Geometry check sheet. Reference: the model listing, model coordinates, mm. Face numbers are marked on the shaded views. A direction names the side the tool comes from. Coordinates: 2 decimals unless noted, no trailing zeros. Loops run counter-clockwise (first coordinate to the right, second up) from the corner with the lowest first, then second, coordinate; pieces in that order, holes last.
from build123d import *

# Parameters (mm, degrees)
SKETCH_1_W          = 30
SKETCH_1_H          = 13
EXTRUDE_1_DEPTH     = 1.4
SKETCH_2_W          = 30
SKETCH_2_H          = 13
EXTRUDE_2_DEPTH     = 4
SKETCH_3_W          = 30
SKETCH_3_H          = 13
EXTRUDE_3_DEPTH     = 1.6
SKETCH_4_W          = 30
SKETCH_4_H          = 8.5
EXTRUDE_4_DEPTH     = 4.5
SKETCH_6_W          = 16.5
SKETCH_6_H          = 7.2
SKETCH_6_W_2        = 15.3
SKETCH_6_H_2        = 6
SKETCH_6_W_3        = 7.5
SKETCH_6_R          = 3
EXTRUDE_5_DEPTH     = 2
SKETCH_7_W          = 10.5
SKETCH_7_H          = 4.5
CUT_EXTRUDE_1_DEPTH = 12
SKETCH_8_W          = 10
SKETCH_8_H          = 1.1
EXTRUDE_6_DEPTH     = 8.05


with BuildPart() as part:
    # Эскиз1 → Бобышка-Вытянуть1 (new body)
    with BuildSketch(Plane.XY):
        with Locations((0, 6.5)):
            Rectangle(SKETCH_1_W, SKETCH_1_H)
    extrude(amount=EXTRUDE_1_DEPTH)

    # Эскиз2 → Бобышка-Вытянуть2 (add)
    with BuildSketch(Plane.XY.offset(1.4)):
        with Locations((0, 6.5)):
            Rectangle(SKETCH_2_W, SKETCH_2_H)
    extrude(amount=EXTRUDE_2_DEPTH)

    # Эскиз3 → Бобышка-Вытянуть3 (add)
    with BuildSketch(Plane.XY.offset(5.4)):
        with Locations((0, 6.5)):
            Rectangle(SKETCH_3_W, SKETCH_3_H)
    extrude(amount=EXTRUDE_3_DEPTH)

    # Эскиз4 → Бобышка-Вытянуть4 (add)
    with BuildSketch(Plane.XY.offset(7)):
        with Locations((0, 6.5)):
            Rectangle(SKETCH_4_W, SKETCH_4_H)
    extrude(amount=EXTRUDE_4_DEPTH)

    # Эскиз6 → Бобышка-Вытянуть5 (add)
    # profile 1 of 2: a face of its own
    with BuildSketch(Plane.XY.offset(11.5)):
        with Locations((5.95, 6.5)):
            Rectangle(SKETCH_6_W, SKETCH_6_H)
        with Locations((5.95, 6.5)):
            Rectangle(SKETCH_6_W_2, SKETCH_6_H_2, mode=Mode.SUBTRACT)
    # profile 2 of 2: a face of its own
    with BuildSketch(Plane.XY.offset(11.5)):
        with Locations((-10.45, 6.5)):
            Rectangle(SKETCH_6_W_3, SKETCH_6_H)
        with Locations((-10.45, 6.5)):
            Circle(SKETCH_6_R, mode=Mode.SUBTRACT)
    extrude(amount=EXTRUDE_5_DEPTH)

    # Эскиз7 → Вырез-Вытянуть1 (cut)
    with BuildSketch(Plane.XY.offset(7)):
        Rectangle(SKETCH_7_W, SKETCH_7_H)
    extrude(amount=-CUT_EXTRUDE_1_DEPTH, mode=Mode.SUBTRACT)

    # Эскиз8 → Бобышка-Вытянуть6 (add)
    with BuildSketch(Plane.XZ.offset(-2.25)):
        with Locations((0, 3.05)):
            Rectangle(SKETCH_8_W, SKETCH_8_H)
    extrude(amount=EXTRUDE_6_DEPTH)


solid = part.part
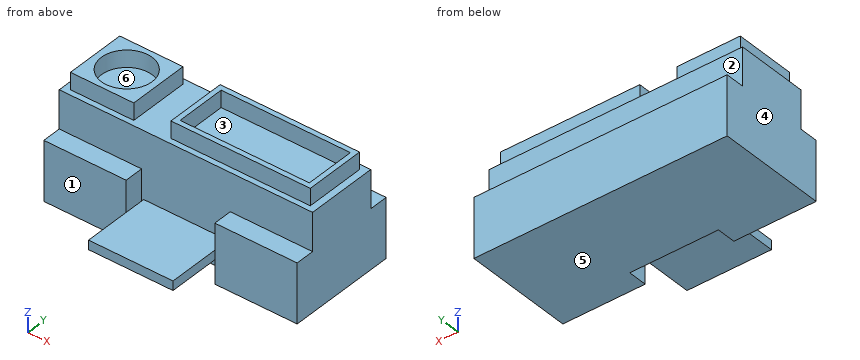
(1) Access from +Z, -Z, +X, -X, +Y, -Y to the whole of each face (thin tool, end or side, straight path). Record for the marked faces 1, 2 and 3.
Findings:
face 1: +Z, -Z, -X, -Y
face 2: +Z, +X, -X, +Y
face 3: +Z
(2) Sectioned sample at B-B on y = 6.5. Record the cut outline in (x, z), and give its area (3 significant figures).
Findings:
outline: (-15, 0) - (15, 0) - (15, 11.5) - (14.2, 11.5) - (14.2, 13.5) - (13.6, 13.5) - (13.6, 11.5) - (-1.7, 11.5) - (-1.7, 13.5) - (-2.3, 13.5) - (-2.3, 11.5) - (-6.7, 11.5) - (-6.7, 13.5) - (-7.45, 13.5) - (-7.45, 11.5) - (-13.45, 11.5) - (-13.45, 13.5) - (-14.2, 13.5) - (-14.2, 11.5) - (-15, 11.5) - close
area: 350 mm2
(3) Sectioned sample at D-D on x = -12.5. Record the cut outline in (y, z).
Findings:
outline: (0, 0) - (13, 0) - (13, 7) - (10.75, 7) - (10.75, 11.5) - (10.1, 11.5) - (10.1, 13.5) - (8.69, 13.5) - (8.69, 11.5) - (4.31, 11.5) - (4.31, 13.5) - (2.9, 13.5) - (2.9, 11.5) - (2.25, 11.5) - (2.25, 7) - (0, 7) - close
(4) Scan lines: L1, parallel to Y at x = -10.45, z = 12.2; L2, parallel to Z at x = -6.25, y = 12; L3, parallel to Z at x = 4.5, y = 10.5. Record each from-to range of solid material in increasing order.
Findings:
L1: y = 2.9 to 3.5, 9.5 to 10.1
L2: z = 0 to 7
L3: z = 0 to 11.5
(5) Gauge pin test, flat ends, axial feed: pin 1 Ø1.6 at (x, z) = (5.5, 12.5) entering from +Y; pin 2 Ø1.5 at (x, y) = (-0.5, 8.5) entering from +Z; pin 3 Ø1.6 at (y, z) = (5, 13) entering from -X. Record the tip position at first contact, or that the pin passes through.
Findings:
pin 1: stops at y = 10.1
pin 2: stops at z = 11.5
pin 3: stops at x = -14.2
(6) Sectioned sample at A-A on z = 6. Record the cut outline in (x, y), and give its area (3 significant figures).
Findings:
outline: (-15, 0) - (-5.25, 0) - (-5.25, 2.25) - (5.25, 2.25) - (5.25, 0) - (15, 0) - (15, 13) - (-15, 13) - close
area: 366 mm2
(7) Sectioned sample at C-C on x = 9.5. Record the cut outline in (y, z), and give its area (3 significant figures).
Findings:
outline: (0, 0) - (13, 0) - (13, 7) - (10.75, 7) - (10.75, 11.5) - (10.1, 11.5) - (10.1, 13.5) - (9.5, 13.5) - (9.5, 11.5) - (3.5, 11.5) - (3.5, 13.5) - (2.9, 13.5) - (2.9, 11.5) - (2.25, 11.5) - (2.25, 7) - (0, 7) - close
area: 132 mm2
(8) Draft check along X on the marked faces 4, 5 and 6. Enter one of: +X half, -X half, draft (parallel to the pull), parting line (faces both ways), or undercut.
Findings:
face 4: -X half
face 5: draft
face 6: undercut
